from build123d import *

# Parameters (mm, degrees)
IZIM1_W                      = 50
IZIM1_H                      = 20
IZIM1_R                      = 1.5
Y_KSEKLIK_EKSTR_ZYON1_DEPTH  = 3.5
IZIM2_W                      = 19.5
IZIM2_H                      = 19.962779687
IZIM2_R                      = 2
Y_KSEKLIK_EKSTR_ZYON2_DEPTH  = 1.5
IZIM4_R                      = 3
KES_EKSTR_ZYON1_DEPTH        = 0.5
IZIM5_W                      = 4.6
IZIM5_H                      = 46.7
Y_KSEKLIK_EKSTR_ZYON3_DEPTH  = 52
IZIM6_W                      = 52
IZIM6_H                      = 4.7
Y_KSEKLIK_EKSTR_ZYON4_DEPTH  = 48
IZIM7_R                      = 2
Y_KSEKLIK_EKSTR_ZYON7_DEPTH  = 1
IZIM8_R                      = 1.5
IZIM8_R_2                    = 11.025
KES_EKSTR_ZYON3_DEPTH        = 67
IZIM9_W                      = 8
IZIM9_H                      = 52.582189456
KES_EKSTR_ZYON4_DEPTH        = 86
IZIM10_W                     = 8
IZIM10_H                     = 54.08264119
KES_EKSTR_ZYON5_DEPTH        = 86
Y_KSEKLIK_EKSTR_ZYON13_DEPTH = 3.5
IZIM13_W                     = 11
IZIM13_H                     = 11.017220313
Y_KSEKLIK_EKSTR_ZYON15_DEPTH = 1.5


with BuildPart() as part:
    # Çizim1 → Yükseklik-Ekstrüzyon1 (new body)
    with BuildSketch(Plane.XY):
        Rectangle(IZIM1_W, IZIM1_H)
        with Locations((-15, 0)):
            Circle(IZIM1_R, mode=Mode.SUBTRACT)
        with Locations((-5, 0)):
            Circle(IZIM1_R, mode=Mode.SUBTRACT)
        with Locations((5, 0)):
            Circle(IZIM1_R, mode=Mode.SUBTRACT)
        with Locations((15, 0)):
            Circle(IZIM1_R, mode=Mode.SUBTRACT)
    extrude(amount=Y_KSEKLIK_EKSTR_ZYON1_DEPTH)

    # Çizim2 → Yükseklik-Ekstrüzyon2 (add)
    with BuildSketch(Plane.ZY.offset(25)):
        with Locations((-6.25, 0.018610156)):
            Rectangle(IZIM2_W, IZIM2_H)
        with Locations((-8.8, 0.496433055)):
            Circle(IZIM2_R, mode=Mode.SUBTRACT)
    extrude(amount=Y_KSEKLIK_EKSTR_ZYON2_DEPTH)

    # Çizim4 → Kes-Ekstrüzyon1 (cut)
    with BuildSketch(Plane.ZY.offset(26.5)):
        with Locations((-8.8, 0.496433055)):
            Circle(IZIM4_R)
    extrude(amount=-KES_EKSTR_ZYON1_DEPTH, mode=Mode.SUBTRACT)

    # Çizim5 → Yükseklik-Ekstrüzyon3 (add)
    with BuildSketch(Plane.ZY.offset(26.5)):
        with Locations((-8.7, 0.02)):
            Rectangle(IZIM5_W, IZIM5_H)
    extrude(amount=Y_KSEKLIK_EKSTR_ZYON3_DEPTH)

    # Çizim6 → Yükseklik-Ekstrüzyon4 (add)
    with BuildSketch(Plane.XY.offset(-6.4)):
        with Locations((-52.5, -20.98)):
            Rectangle(IZIM6_W, IZIM6_H)
    extrude(amount=Y_KSEKLIK_EKSTR_ZYON4_DEPTH)

    # Çizim7 → Yükseklik-Ekstrüzyon7 (add)
    with BuildSketch(Plane(origin=(-25, 0, 0), x_dir=(0, 0, -1), z_dir=(1, 0, 0))):
        with Locations((8.8, 0.496433055)):
            Circle(IZIM7_R)
    extrude(amount=-Y_KSEKLIK_EKSTR_ZYON7_DEPTH)

    # Çizim8 → Kes-Ekstrüzyon3 (cut)
    with BuildSketch(Plane.XY.offset(-6.4)):
        with Locations((-31.9, -13.23)):
            Circle(IZIM8_R)
        with Locations((-63.25, -13.23)):
            Circle(IZIM8_R)
        with Locations((-31.9, 17.97)):
            Circle(IZIM8_R)
        with Locations((-63.25, 17.97)):
            Circle(IZIM8_R)
        with Locations((-47.575, 2.37)):
            Circle(IZIM8_R_2)
    extrude(amount=-KES_EKSTR_ZYON3_DEPTH, mode=Mode.SUBTRACT)

    # Çizim9 → Kes-Ekstrüzyon4 (cut)
    with BuildSketch(Plane.XY.offset(-6.4)):
        with Locations((-74.5, -2.921094728)):
            Rectangle(IZIM9_W, IZIM9_H)
    extrude(amount=KES_EKSTR_ZYON4_DEPTH, mode=Mode.SUBTRACT)

    # Çizim10 → Kes-Ekstrüzyon5 (cut)
    with BuildSketch(Plane.XY.offset(-6.4)):
        with Locations((-74.5, -3.671320595)):
            Rectangle(IZIM10_W, IZIM10_H)
    extrude(amount=-KES_EKSTR_ZYON5_DEPTH, mode=Mode.SUBTRACT)

    # Çizim12 → Yükseklik-Ekstrüzyon13 (add)
    with BuildSketch(Plane.XY.offset(3.5)):
        Polygon((-26.5, -20.98), (-26.5, -5.633173316), (5.348461145, -5.633173316), align=None)
    extrude(amount=-Y_KSEKLIK_EKSTR_ZYON13_DEPTH)

    # Çizim13 → Yükseklik-Ekstrüzyon15 (add)
    with BuildSketch(Plane(origin=(-26.5, 0, 0), x_dir=(0, 0, -1), z_dir=(1, 0, 0))):
        with Locations((5.5, -15.471389844)):
            Rectangle(IZIM13_W, IZIM13_H)
    extrude(amount=Y_KSEKLIK_EKSTR_ZYON15_DEPTH)


solid = part.part
Model file for the job. Use its own axes, mm. A direction names the side the tool comes from. Give positions to 0.01 mm unless a question says otherwise; leave off trailing zeros. Loops run counter-clockwise (first coordinate to the right, second up) from the corner with the lowest first, then second, coordinate; pieces in that order, holes last. Notation, with made-up numbers: (21.5, 35.5) -> (69.5, 35.5) arc R7 cw to (69.5, 45.5) -> close; hole circle Ø7 at (61.5, 86). An arc over 180 degrees is marked (long way). Use a Markdown table: item, result. Add a question column.
(1) Slice it at B-B on x = -31.9. List the corners of the cut face in (y, z).
(2) Slice it at D-D on y = 17.97. List the corners of the cut face in (x, z), and give its area (3 significant figures).
(3) Slice it at C-C on z = -8.8. List the corners of the cut face in (x, y) (3 decimals).
(4) Tool access for faces 1 (the flat face through (10, -10, 2)), 2 (the flat face through (-26, 1, -9)), 3 (the flat face through (-49, -18.63, 17)), 4 (the flat face through (0, -2, 0)), 5 (the cylindrical face through (-61.864, -13.805, -8.668)): list every direction of +Z, -Z, +X, -X, +Y, -Y with a clear straight run to the whole face (end or side of a thin tool).
(5) Slice it at A-A on x = 15. List the corners of the cut face in (y, z).
(6) Mould opens along X. For faces 6 (the flat face through (-48, -11, -11)), 7 (the flat face through (-14.947, -15.413, 1.774)), 8 (the cylindrical face through (-26.254, -0.653, -6.029)), 9 (the cylindrical face through (13.5, 0.07, 1.73)) say: +X half, -X half, draft (parallel to the pull), parting line (faces both ways), or undercut.
(7) Drop flat-ended pins along their axis: pin 1 Ø1.5 at (x, y) = (-25.5, 8) entering from +Z; pin 2 Ø24 at (x, y) = (-3.5, -5.5) entering from -Z; pin 3 Ø8 at (y, z) = (0.5, -2) entering from -X. Give the stop position or say it passes through.
(8) Wall check: line 1 along Y through (x, z) = (-63, -7); line 2 along Y through (x, z) = (-31.9, -8.2); line 3 along Y through (x, z) = (-47, -8). Give the ranges that are in metal, low to high.
Filled sheet:
| question | item | result |
|---|---|---|
| 1 | outline | (-23.33, -11) -> (-14.73, -11) -> (-14.73, -6.4) -> (-18.63, -6.4) -> (-18.63, 41.6) -> (-23.33, 41.6) -> close; (-11.73, -11) -> (16.47, -11) -> (16.47, -6.4) -> (-11.73, -6.4) -> close; (19.47, -11) -> (23.37, -11) -> (23.37, -6.4) -> (19.47, -6.4) -> close |
| 2 | outline | (-70.5, -11) -> (-64.75, -11) -> (-64.75, -6.4) -> (-70.5, -6.4) -> close; (-61.75, -11) -> (-33.4, -11) -> (-33.4, -6.4) -> (-61.75, -6.4) -> close; (-30.4, -11) -> (-26.5, -11) -> (-26.5, -6.4) -> (-30.4, -6.4) -> close |
| 2 | area | 175 mm2 |
| 3 | outline | (-70.5, -23.33) -> (-26.5, -23.33) -> (-26.5, -20.98) -> (-25, -20.98) -> (-25, 10) -> (-26.5, 10) -> (-26.5, 23.37) -> (-70.5, 23.37) -> close; hole circle Ø3 at (-63.25, -13.23); hole circle Ø3 at (-63.25, 17.97); hole circle Ø22.05 at (-47.575, 2.37); hole circle Ø3 at (-31.9, -13.23); hole circle Ø3 at (-31.9, 17.97); hole (-26.5, -2.504) -> (-26, -2.504) -> (-26, 3.496) -> (-26.5, 3.496) -> close |
| 4 | face 1 | +Z, -Z, +X, -Y |
| 4 | face 2 | none |
| 4 | face 3 | +Z, -X, +Y |
| 4 | face 4 | -Z, +X, +Y, -Y |
| 4 | face 5 | +Z, -Z |
| 5 | outline | (-10, 0) -> (-1.5, 0) -> (-1.5, 3.5) -> (-10, 3.5) -> close; (1.5, 0) -> (10, 0) -> (10, 3.5) -> (1.5, 3.5) -> close |
| 6 | face 6 | draft |
| 6 | face 7 | +X half |
| 6 | face 8 | undercut |
| 6 | face 9 | undercut |
| 7 | pin 1 | z = 3.5 |
| 7 | pin 2 | z = 0 |
| 7 | pin 3 | x = -26.5 |
| 8 | line 1 | -23.33 to -14.71, -11.75 to 16.49, 19.45 to 23.37 |
| 8 | line 2 | -23.33 to -14.73, -11.73 to 16.47, 19.47 to 23.37 |
| 8 | line 3 | -23.33 to -8.64, 13.38 to 23.37 |
